Autodesk Inventor part; units mm, degrees
ref_plane "YZ Plane" through (0, 0, 0) normal (1, 0, 0) x (0, 1, 0)
ref_plane "XZ Plane" through (0, 0, 0) normal (0, 1, 0) x (-1, 0, 0)
ref_plane "XY Plane" through (0, 0, 0) normal (0, 0, 1) x (1, 0, 0)
sketch "スケッチ1" plane through (0, 0, 0) normal (0, 0, 1) x (1, 0, 0)
  line L0 (0, 0) -> (41, 0)
  line L1 (41, 0) -> (41, -21)
  line L2 (41, -21) -> (0, -21)
  line L3 (0, -21) -> (0, 0)
  dimension "d0" = 41
  dimension "d1" = 21
extrude "押し出し1" add sketch "スケッチ1" along normal blind 30.5
sketch "スケッチ2" plane through (0, 0, 0) normal (0, 0, -1) x (-1, 0, 0)
  line L0 (0, 0) -> (-41, 0)
  line L1 (0, -21) -> (0, 0)
  line L2 (-41, 0) -> (-41, -21)
  line L3 (0, -21) -> (-41, -21)
  point P0 (-2.5, -2.5)
  point P1 (-38.5, -2.5)
  point P2 (-2.5, -18.5)
  point P3 (-38.5, -18.5)
  dimension "d32" = 16
  dimension "d33" = 2.5
  dimension "d34" = 36
  dimension "d35" = 2.5
  dimension "d36" = 2.5
  dimension "d37" = 36
  dimension "d39" = 16
  dimension "d40" = 2.5
hole "穴1" at (2.5, -2.5, 0) at (38.5, -2.5, 0) at (2.5, -18.5, 0) at (38.5, -18.5, 0) direction (0, 0, 1) diameter 2 end through all
sketch "スケッチ3" plane through (0, 0, 0) normal (0, 0, -1) x (-1, 0, 0)
  circle A0 centre (-10.25, -10.5) radius 5.5
  point P0 (0, 0)
  dimension "d11" = 11
extrude "押し出し2" add sketch "スケッチ3" along normal blind 1
sketch "スケッチ4" plane through (10.25, -10.5, -1) normal (0, 0, -1) x (-1, 0, 0)
  circle A0 centre (0, 0) radius 1.5
  point P0 (10.25, 10.5)
  dimension "d14" = 3
extrude "押し出し3" cut sketch "スケッチ4" against normal blind 40
sketch "スケッチ5" plane through (10.25, -10.5, -1) normal (0, 0, -1) x (-1, 0, 0)
  circle A0 centre (0, 0) radius 2
  point P0 (10.25, 10.5)
  dimension "d17" = 4
extrude "押し出し4" add sketch "スケッチ5" along normal blind 3
sketch "スケッチ6" plane through (10.25, -10.5, -4) normal (0, 0, -1) x (-1, 0, 0)
  circle A0 centre (0, 0) radius 1.5
  point P0 (10.25, 10.5)
  dimension "d20" = 3
extrude "押し出し5" cut sketch "スケッチ6" against normal blind 4
sketch "スケッチ8" plane through (0, 0, 30.5) normal (0, 0, 1) x (1, 0, 0)
  circle A0 centre (10.25, -10.5) radius 5.5
  point P0 (0, 0)
  dimension "d23" = 11
extrude "押し出し6" add sketch "スケッチ8" along normal blind 1
sketch "スケッチ9" plane through (10.25, -10.5, 31.5) normal (0, 0, 1) x (1, 0, 0)
  circle A0 centre (0, 0) radius 1.5
  circle A1 centre (0, 0) radius 2
  point P0 (-10.25, 10.5)
  dimension "d26" = 4
extrude "押し出し7" add sketch "スケッチ9" along normal blind 3
sketch "スケッチ10" plane through (10.25, -10.5, 31.5) normal (0, 0, 1) x (1, 0, 0)
  circle A0 centre (0, 0) radius 1.5
  point P0 (-10.25, 10.5)
  dimension "d29" = 3
extrude "押し出し8" cut sketch "スケッチ10" against normal blind 3
properties part number "KRS-2542HV ICS" material "PVC、軟質"
Read the model definition and answer for the solid it produces. Units are mm, in the model's axes. A direction names the side the tool comes from. Coordinates: 2 decimals unless noted, no trailing zeros. Write each loop counter-clockwise with the first axis right and the second up, starting at its lowest first coordinate (ties: lowest second). Pieces come first, ordered by that corner, then holes. Notation, with made-up numbers: (-3.75, 38.5) - (49.25, 38.5) arc R9 ccw to (49.25, 53.5) - close; hole circle Ø11 at (62.5, -16.5). An arc over 180 degrees is marked (long way). Answer as a JSON object with one key per item and string values. Group by question number.
1. A cutting plane is placed at B-B (x = 38.5). Determine the outline of the cut face in (y, z).
2. The mould has two halves that part along Y. Classify faces 1 (the cylindrical face through (37.51, -2.63, 15.46)), 2 (the flat face through (41, -10, 15)), 3 (the cylindrical face through (37.51, -18.63, 15.46)), 4 (the flat face through (20, 0, 15)): +Y half, -Y half, draft (parallel to the pull), parting line (faces both ways), or undercut.
3. A cutting plane is placed at D-D (y = -18.5). Determine the outline of the cut face in (x, z), plus the area to 3 significant figures.
4. A cutting plane is placed at A-A (x = 10.25). Determine the outline of the cut face in (y, z), plus the area to 3 significant figures.
5. Which of the six approach directions +Z, -Z, +X, -X, +Y, -Y give full straight-line access (tool end or side, diameter ignored) to faces 5 (the cylindrical face through (9.99, -12.483, 32.979)), 6 (the cylindrical face through (10.51, -12.483, -2.479)), 7 (the flat face through (0, -11, 15))?
6. Each of these flat-tipped pins is pushed along its axis until it touches: P1, Ø2, axis at x = 7.5, z = 1, coming from the +Y side; P2, Ø2.5, axis at x = 38.5, y = -2.5, coming from the +Z side; P3, Ø6.5, axis at x = 19.5, y = -10, coming from the -Z side; P4, Ø3, axis at x = 5, y = -14, coming from the -Z side. Where does it stop, or does it pass through?
7. Consider L1, parallel to Y at x = 2.5, z = 18.5; L2, parallel to X at y = -2.5, z = 7.5; L3, parallel to Z at x = 34, y = -3. Determine where each line is inside the solid, lowest interval first. Write a range as [from, to].
8. A cutting plane is placed at C-C (y = -10.5). Determine the outline of the cut face in (x, z).
Worked out:
{
 "1": {"outline": "(-21, 0) - (-19.5, 0) - (-19.5, 30.5) - (-21, 30.5) - close; (-17.5, 0) - (-3.5, 0) - (-3.5, 30.5) - (-17.5, 30.5) - close; (-1.5, 0) - (0, 0) - (0, 30.5) - (-1.5, 30.5) - close"},
 "2": {"face 1": "undercut", "face 2": "draft", "face 3": "undercut", "face 4": "+Y half"},
 "3": {"outline": "(0, 0) - (1.5, 0) - (1.5, 30.5) - (0, 30.5) - close; (3.5, 0) - (37.5, 0) - (37.5, 30.5) - (3.5, 30.5) - close; (39.5, 0) - (41, 0) - (41, 30.5) - (39.5, 30.5) - close", "area": "1,130 mm²"},
 "4": {"outline": "(-21, 0) - (-16, 0) - (-16, -1) - (-12.5, -1) - (-12.5, -4) - (-12, -4) - (-12, 34.5) - (-12.5, 34.5) - (-12.5, 31.5) - (-16, 31.5) - (-16, 30.5) - (-21, 30.5) - close; (-9, -4) - (-8.5, -4) - (-8.5, -1) - (-5, -1) - (-5, 0) - (0, 0) - (0, 30.5) - (-5, 30.5) - (-5, 31.5) - (-8.5, 31.5) - (-8.5, 34.5) - (-9, 34.5) - close", "area": "571 mm²"},
 "5": {"face 5": "+Z", "face 6": "-Z", "face 7": "+Z, -Z, -X, +Y, -Y"},
 "6": {"P1": "stops at y = 0", "P2": "stops at z = 30.5", "P3": "stops at z = 0", "P4": "stops at z = -1"},
 "7": {"L1": "y = [-21, -19.5], [-17.5, -3.5], [-1.5, 0]", "L2": "x = [0, 1.5], [3.5, 37.5], [39.5, 41]", "L3": "z = [0, 30.5]"},
 "8": {"outline": "(0, 0) - (4.75, 0) - (4.75, -1) - (8.25, -1) - (8.25, -4) - (8.75, -4) - (8.75, 34.5) - (8.25, 34.5) - (8.25, 31.5) - (4.75, 31.5) - (4.75, 30.5) - (0, 30.5) - close; (11.75, -4) - (12.25, -4) - (12.25, -1) - (15.75, -1) - (15.75, 0) - (41, 0) - (41, 30.5) - (15.75, 30.5) - (15.75, 31.5) - (12.25, 31.5) - (12.25, 34.5) - (11.75, 34.5) - close"}
}
